For this review, take the finished solid that the model builds, in its own axes (mm). Face numbers are marked on the shaded views. A direction names the side the tool comes from. Give positions to 0.01 mm unless a question says otherwise; leave off trailing zeros. Order: outer loops, then holes, each group sorted by start corner. A loop starts at its lowest first (then second) coordinate and runs counter-clockwise, first axis right, second up.
Item 1: For probe 1 along X at (y, z) = (11.5, -14); probe 2 along Z at (x, y) = (-4, 38); probe 3 along Y at (x, z) = (49, -8.5), list the stretches that pass through material, from the lowest coordinate up.
Item 2: For P1, Ø12.5, axis at x = -5, y = 10, coming from the +Z side; P2, Ø10, axis at x = 57.5, z = -27, coming from the +Y side; P3, Ø0.7, axis at y = 0.5, z = -16.5, coming from the -X side, all flat-tipped, find the tip position at first contact; note any pin that passes through.
Item 3: Consider section D-D (x = 55). Give the boundary of the cut face in (y, z), plus the area to 3 significant figures.
Item 4: The part is to be moulded in two halves that separate along X. For the marked faces 6, 7, 8 and 9, say which applies: released by +X, released by -X, zero draft, split by the parting line, or undercut.
Item 5: Consider section C-C (z = -5). Give the boundary of the cut face in (x, y), plus the area to 3 significant figures.
Item 6: Machinability: for the marked faces 1, 2, 3, 4 and 5, which of the approach directions +Z, -Z, +X, -X, +Y, -Y give a long, thin tool a straight path to every point of the face, cutting with its end or side? Answer none if there is none.
Item 7: Consider section A-A (y = 23). Give the boundary of the cut face in (x, z), plus the area to 3 significant figures.
Item 8: Consider section B-B (x = 7.5). Give the boundary of the cut face in (y, z).
```python
from build123d import *

# Parameters (mm, degrees)
BOSS_EXTRUDE1_DEPTH = 38.1
CUT_EXTRUDE1_DEPTH  = 2.54
CUT_EXTRUDE2_DEPTH  = 34.29
BOSS_EXTRUDE2_DEPTH = 25.4


with BuildPart() as part:
    # Sketch1 → Boss-Extrude1 (new body)
    with BuildSketch(Plane(origin=(0, 0, 0), x_dir=(1, 0, 0), z_dir=(0, 1, 0))):
        Polygon((12.853808955, 0.174987325), (12.853808955, 37.417012675), (82.296, 25.146), (82.296, 12.446), align=None)
    extrude(amount=BOSS_EXTRUDE1_DEPTH)

    # Sketch3 → Cut-Extrude1 (cut)
    with BuildSketch(Plane(origin=(0, 35.56, 0), x_dir=(1, 0, 0), z_dir=(0, 1, 0))):
        Polygon((79.756, 14.576512841), (79.756, 23.015487159), (15.393808955, 34.388821586), (15.393808955, 3.203178414), align=None)
    extrude(amount=CUT_EXTRUDE1_DEPTH, mode=Mode.SUBTRACT)

    # Sketch6 → Cut-Extrude2 (cut)
    with BuildSketch(Plane(origin=(0, 35.56, 0), x_dir=(1, 0, 0), z_dir=(0, 1, 0))):
        Polygon((81.026, 13.511256421), (81.026, 24.080743579), (14.123808955, 35.90291713), (14.123808955, 1.68908287), align=None)
    extrude(amount=-CUT_EXTRUDE2_DEPTH, mode=Mode.SUBTRACT)

    # Sketch8 → Boss-Extrude2 (add)
    with BuildSketch(Plane.ZY.offset(-12.853808955)):
        Polygon((-31.26502256, 38.1), (-31.26502256, 0), (-18.796, 2.1986251), (-6.32697744, 0), (-6.32697744, 38.1), (-18.796, 40.2986251), align=None)
    extrude(amount=BOSS_EXTRUDE2_DEPTH)


solid = part.part
```
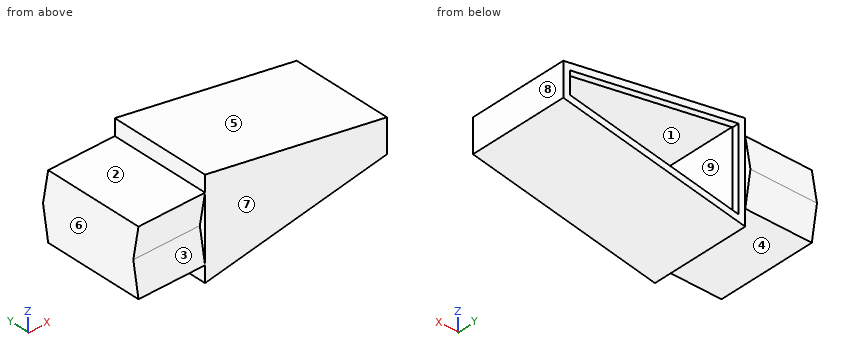
Resolved:
1. probe 1: x = -12.55 to 14.12, 81.03 to 82.3
1. probe 2: z = -31.27 to -6.33
1. probe 3: y = 0 to 1.27, 35.56 to 38.1
2. P1: stops at z = -6.33
2. P2: stops at y = 38.1
2. P3: stops at x = 12.85
3. outline: (0, -29.97) - (38.1, -29.97) - (38.1, -27.39) - (35.56, -27.39) - (35.56, -28.68) - (1.27, -28.68) - (1.27, -8.91) - (35.56, -8.91) - (35.56, -10.2) - (38.1, -10.2) - (38.1, -7.62) - (0, -7.62) - close
3. area: 130 mm2
4. face 6: released by -X
4. face 7: zero draft
4. face 8: released by +X
4. face 9: undercut
5. outline: (12.85, 0) - (40.16, 0) - (40.16, 38.1) - (25.56, 38.1) - (25.56, 35.56) - (32.86, 35.56) - (32.86, 1.27) - (14.12, 1.27) - (14.12, 35.56) - (15.39, 35.56) - (15.39, 38.1) - (12.85, 38.1) - close
5. area: 372 mm2
6. face 1: none
6. face 2: +Z, -X, +Y, -Y
6. face 3: -X, -Y
6. face 4: -Z, -X, +Y, -Y
6. face 5: +Z, +X, +Y, -Y
7. outline: (-12.55, -31.27) - (12.85, -31.27) - (12.85, -37.42) - (82.3, -25.15) - (82.3, -12.45) - (12.85, -0.17) - (12.85, -6.33) - (-12.55, -6.33) - close; hole (14.12, -35.9) - (81.03, -24.08) - (81.03, -13.51) - (14.12, -1.69) - close
7. area: 869 mm2
8. outline: (0, -31.27) - (38.1, -31.27) - (40.3, -18.8) - (38.1, -6.33) - (0, -6.33) - (2.2, -18.8) - close
